Verification items for the finished model (mm, model axes). A direction names the side the tool comes from. Round coordinates to 2 decimals unless told otherwise and drop trailing zeros. Write each loop counter-clockwise with the first axis right and the second up, starting at its lowest first coordinate (ties: lowest second). Pieces come first, ordered by that corner, then holes. Notation, with made-up numbers: (11, 9) - (61, 9) arc R32 ccw to (61, 39) - close; hole circle Ø3 at (10, 11.5). An arc over 180 degrees is marked (long way). Write each question's results on one line, items separated by ' | '.
```python
from build123d import *

# Parameters (mm, degrees)
SKETCH1_R           = 12
BOSS_EXTRUDE1_DEPTH = 1.5
SKETCH2_R           = 3.25
BOSS_EXTRUDE2_DEPTH = 2
SKETCH3_R           = 2.5
CUT_EXTRUDE1_DEPTH  = 18.327723451
SKETCH5_R           = 0.75
CUT_EXTRUDE3_DEPTH  = 2


with BuildPart() as part:
    # Sketch1 → Boss-Extrude1 (new body)
    with BuildSketch(Plane(origin=(0, 0, 0), x_dir=(1, 0, 0), z_dir=(0, 1, 0))):
        with Locations(Location((0, 0, 0), (0, 0, 270))):
            Circle(SKETCH1_R)
    extrude(amount=BOSS_EXTRUDE1_DEPTH)

    # Sketch2 → Boss-Extrude2 (add)
    with BuildSketch(Plane(origin=(0, 1.5, 0), x_dir=(1, 0, 0), z_dir=(0, 1, 0))):
        with Locations(Location((0, 0, 0), (0, 0, 270))):
            Circle(SKETCH2_R)
    extrude(amount=BOSS_EXTRUDE2_DEPTH)

    # Sketch3 → Cut-Extrude1 (cut, through all)
    with BuildSketch(Plane(origin=(0, 3.5, 0), x_dir=(1, 0, 0), z_dir=(0, 1, 0))):
        with Locations(Location((0, 0, 0), (0, 0, 270))):
            Circle(SKETCH3_R)
    extrude(amount=-CUT_EXTRUDE1_DEPTH, mode=Mode.SUBTRACT)

    # Sketch5 → Cut-Extrude3 (cut)
    with BuildSketch(Plane(origin=(0, 1.5, 0), x_dir=(1, 0, 0), z_dir=(0, 1, 0))):
        with Locations(Location((0, 7.5, 0), (0, 0, 270))):
            Circle(SKETCH5_R)
        with Locations(Location((5.303300859, 5.303300859, 0), (0, 0, 270))):
            Circle(SKETCH5_R)
        with Locations(Location((7.5, 0, 0), (0, 0, 270))):
            Circle(SKETCH5_R)
        with Locations(Location((5.303300859, -5.303300859, 0), (0, 0, 270))):
            Circle(SKETCH5_R)
        with Locations(Location((0, -7.5, 0), (0, 0, 270))):
            Circle(SKETCH5_R)
        with Locations(Location((-5.303300859, -5.303300859, 0), (0, 0, 270))):
            Circle(SKETCH5_R)
        with Locations(Location((-7.5, 0, 0), (0, 0, 270))):
            Circle(SKETCH5_R)
        with Locations(Location((-5.303300859, 5.303300859, 0), (0, 0, 270))):
            Circle(SKETCH5_R)
    extrude(amount=-CUT_EXTRUDE3_DEPTH, mode=Mode.SUBTRACT)


solid = part.part
```
(1) Thickness scan on L1, parallel to X at y = 0.85, z = 0; L2, parallel to X at y = 2.7, z = 0; L3, parallel to Y at x = 10.25, z = 3.25. Record the ranges inside material, lowest first.
Answer:
L1: -12 to -8.25, -6.75 to -2.5, 2.5 to 6.75, 8.25 to 12 | L2: -3.25 to -2.5, 2.5 to 3.25 | L3: 0 to 1.5
(2) Section check D-D (x = 7.5). Record the cut outline in (y, z).
Answer:
outline: (0, -9.37) - (1.5, -9.37) - (1.5, -0.75) - (0, -0.75) - close; (0, 0.75) - (1.5, 0.75) - (1.5, 9.37) - (0, 9.37) - close
(3) Section check B-B (z = 0). Record the cut outline in (x, y), plus the area to 3 significant figures.
Answer:
outline: (-12, 0) - (-8.25, 0) - (-8.25, 1.5) - (-12, 1.5) - close; (-6.75, 0) - (-2.5, 0) - (-2.5, 3.5) - (-3.25, 3.5) - (-3.25, 1.5) - (-6.75, 1.5) - close; (2.5, 0) - (6.75, 0) - (6.75, 1.5) - (3.25, 1.5) - (3.25, 3.5) - (2.5, 3.5) - close; (8.25, 0) - (12, 0) - (12, 1.5) - (8.25, 1.5) - close | area: 27.0 mm2
(4) Mould release check, pull along X, two halves, no side actions. Record for faces 3 (the flat face through (-2.5, 1.5, 2.5)), 4 (the cylindrical face through (3.604, 0.74, 11.446)), 5 (the cylindrical face through (0.03, 0.76, 6.75)): released by +X, released by -X, zero draft, split by the parting line, or undercut.
Answer:
face 3: zero draft | face 4: split by the parting line | face 5: undercut
(5) Section check A-A (x = 0). Record the cut outline in (y, z), plus the area to 3 significant figures.
Answer:
outline: (0, -12) - (1.5, -12) - (1.5, -8.25) - (0, -8.25) - close; (0, -6.75) - (1.5, -6.75) - (1.5, -3.25) - (3.5, -3.25) - (3.5, -2.5) - (0, -2.5) - close; (0, 2.5) - (3.5, 2.5) - (3.5, 3.25) - (1.5, 3.25) - (1.5, 6.75) - (0, 6.75) - close; (0, 8.25) - (1.5, 8.25) - (1.5, 12) - (0, 12) - close | area: 27.0 mm2
(6) Set-up check for faces 1 (the cylindrical face through (-1.978, 2.486, -2.579)), 2 (the cylindrical face through (-2.44, 1.77, -0.54)): record each of +Z, -Z, +X, -X, +Y, -Y from which the full face is reachable in a straight line by a thin tool's end or side.
Answer:
face 1: +Y | face 2: +Y, -Y
(7) Go/stop test with flat-tipped pins: pin 1 Ø1 at (y, z) = (3, -7.5) entering from +X; pin 2 Ø1 at (y, z) = (1, 3) entering from +X; pin 3 Ø1.5 at (y, z) = (1.5, -4.5) entering from +X. Record where each tip stops, or that it passes through.
Answer:
pin 1: through | pin 2: x = 11.74 | pin 3: x = 11.4
(8) Section check C-C (y = 1). State how many separate pieces and enclosed holes the cut face has, plus the area to 3 significant figures.
Answer:
separate pieces: 1 | enclosed holes: 9 | area: 419 mm2
